For this review, take the finished solid that the model builds, in its own axes (mm). A direction names the side the tool comes from. Coordinates: 2 decimals unless noted, no trailing zeros. Loops run counter-clockwise (first coordinate to the right, second up) from the corner with the lowest first, then second, coordinate; pieces in that order, holes last. Notation, with made-up numbers: (15.25, 49.5) - (23.25, 49.5) arc R17 ccw to (23.25, 65.5) - close; hole circle Ø3 at (21.25, 9.5). An arc over 180 degrees is marked (long way). Answer as a JSON object with one key per item and string values. Group by question number.
Item 1: Mouldability with a two-part tool opening along Y and no side actions: class faces 1 (the flat face through (-19, -17, 0)), 2 (the cylindrical face through (-14.93, 28.966, 5.521)), 3 (the cylindrical face through (-14.93, -2.85, 13.01)) as released by +Y, released by -Y, zero draft, split by the parting line, or undercut.
Item 2: Clearance check with flat-ended pins moving along their axes: pin 1 (10.5 mm diameter, centred on x = -15, y = -20, fed in from -Z); pin 2 (3 mm diameter, centred on x = -12.5, z = -4, fed in from -Y); pin 3 (1.5 mm diameter, centred on x = -25, z = 2, fed in from +Y). State where each tip first meets the part, or that it passes through.
Item 3: We need section A-A (z = 5). State how many separate pieces and enclosed holes the cut face has, then the cut area to 3 significant figures.
Item 4: We need section D-D (y = 4). Give the boundary of the cut face in (x, z).
Item 5: We need section B-B (y = -20). Give the boundary of the cut face in (x, z), then the cut area to 3 significant figures.
Item 6: Tool access review of faces 4 (the flat face through (-20, 17, 5)), 5 (the flat face through (-10, 17, 5)), 6 (the flat face through (-19, -17, 10)): name each direction out of +Z, -Z, +X, -X, +Y, -Y from which nothing blocks a thin tool from reaching the whole face with its end or side.
Item 7: To check wall thickness, follow line 1 (Y direction, x = -15, z = 5.25); line 2 (X direction, y = -20, z = 3.75); line 3 (Y direction, x = -15, z = 3). State the ranges of each line that lie inside material, in increasing order.
from build123d import *

# Parameters (mm, degrees)
SKETCH1_W           = 30
SKETCH1_H           = 35
BOSS_EXTRUDE1_DEPTH = 10
FILLET1_R           = 10
FILLET2_R           = 10
SKETCH11_R          = 4
CUT_EXTRUDE3_DEPTH  = 14
SKETCH12_W          = 10
SKETCH12_H          = 30
BOSS_EXTRUDE4_DEPTH = 35
SKETCH15_R          = 4
CUT_EXTRUDE4_DEPTH  = 35
FILLET10_R          = 10
FILLET11_R          = 10
FILLET13_R          = 10
FILLET14_R          = 10
FILLET15_R          = 10
FILLET16_R          = 10


with BuildPart() as part:
    # Sketch1 → Boss-Extrude1 (new body)
    with BuildSketch(Plane.XY):
        with Locations((-15, -17.5)):
            Rectangle(SKETCH1_W, SKETCH1_H)
    extrude(amount=BOSS_EXTRUDE1_DEPTH)

    # Fillet1
    fillet1_edges = [part.edges().sort_by_distance(p)[0] for p in [
        (-30, -35, 5),
    ]]
    fillet(fillet1_edges, radius=FILLET1_R)

    # Fillet2
    fillet2_edges = [part.edges().sort_by_distance(p)[0] for p in [
        (0, -35, 5),
    ]]
    fillet(fillet2_edges, radius=FILLET2_R)

    # Sketch11 → Cut-Extrude3 (cut)
    with BuildSketch(Plane.XY):
        with Locations(Location((-15, -20, 0), (0, 0, 180))):
            Circle(SKETCH11_R)
    extrude(amount=CUT_EXTRUDE3_DEPTH, mode=Mode.SUBTRACT)

    # Sketch12 → Boss-Extrude4 (add)
    with BuildSketch(Plane(origin=(0, 0, 0), x_dir=(1, 0, 0), z_dir=(0, 1, 0))):
        with Locations((-15, -5)):
            Rectangle(SKETCH12_W, SKETCH12_H)
    extrude(amount=BOSS_EXTRUDE4_DEPTH)

    # Sketch15 → Cut-Extrude4 (cut)
    with BuildSketch(Plane(origin=(-10, 0, 0), x_dir=(0, 0, -1), z_dir=(1, 0, 0))):
        with Locations((-5, 25)):
            Circle(SKETCH15_R)
    extrude(amount=-CUT_EXTRUDE4_DEPTH, mode=Mode.SUBTRACT)

    # Fillet10
    fillet10_edges = [part.edges().sort_by_distance(p)[0] for p in [
        (-15, 35, -10),
    ]]
    fillet(fillet10_edges, radius=FILLET10_R)

    # Fillet11
    fillet11_edges = [part.edges().sort_by_distance(p)[0] for p in [
        (-15, 35, 20),
    ]]
    fillet(fillet11_edges, radius=FILLET11_R)

    # Fillet13
    fillet13_edges = [part.edges().sort_by_distance(p)[0] for p in [
        (-15, 0, 10),
    ]]
    fillet(fillet13_edges, radius=FILLET13_R - 0.0001)  # a hair under: the kernel refuses the full size

    # Fillet14
    fillet14_edges = [part.edges().sort_by_distance(p)[0] for p in [
        (-15, 0, 0),
    ]]
    fillet(fillet14_edges, radius=FILLET14_R - 0.0001)  # a hair under: the kernel refuses the full size

    # Fillet15
    fillet15_edges = [part.edges().sort_by_distance(p)[0] for p in [
        (-10, 0, 5),
    ]]
    fillet(fillet15_edges, radius=FILLET15_R - 0.0001)  # a hair under: the kernel refuses the full size

    # Fillet16
    fillet16_edges = [part.edges().sort_by_distance(p)[0] for p in [
        (-20, 0, 5),
    ]]
    fillet(fillet16_edges, radius=FILLET16_R - 0.0001)  # a hair under: the kernel refuses the full size


solid = part.part
Check sheet entries:
{
 "1": {"face 1": "zero draft", "face 2": "undercut", "face 3": "released by -Y"},
 "2": {"pin 1": "stops at z = 0", "pin 2": "stops at y = -3.39", "pin 3": "stops at y = 1.82"},
 "3": {"separate pieces": "2", "enclosed holes": "1", "area": "1,270 mm2"},
 "4": {"outline": "(-22, 0) - (-20, 0) - (-20, -10) - (-10, -10) - (-10, 0) - (-8, 0) - (-8, 10) - (-10, 10) - (-10, 20) - (-20, 20) - (-20, 10) - (-22, 10) - close"},
 "5": {"outline": "(-30, 0) - (-19, 0) - (-19, 10) - (-30, 10) - close; (-11, 0) - (0, 0) - (0, 10) - (-11, 10) - close", "area": "220 mm2"},
 "6": {"face 4": "-X, +Y", "face 5": "+X, +Y", "face 6": "+Z, -Y"},
 "7": {"line 1": "y = -35 to -24, -16 to 21.01, 28.99 to 35", "line 2": "x = -30 to -19, -11 to 0", "line 3": "y = -35 to -24, -16 to 21.54, 28.46 to 35"}
}
